Part model, mm, in its own coordinate system. A direction names the side the tool comes from. Coordinates: 2 decimals unless noted, no trailing zeros. Loops run counter-clockwise (first coordinate to the right, second up) from the corner with the lowest first, then second, coordinate; pieces in that order, holes last. Notation, with made-up numbers: (53.5, 42) -> (106.5, 42) arc R4 ccw to (106.5, 46) -> close; hole circle Ø4 at (0, 74.5). An arc over 180 degrees is marked (long way). Use one line per item in the form item = value. Start each with the question number.
(1) Drill centre lines: L1, parallel to Z at x = 0.85, y = 5; L2, parallel to Y at x = 2.6, z = -13 (3 decimals); L3, parallel to Y at x = 0.2, z = -29 (3 decimals). Where is each one in solid material? Low to high. Write a range as [from, to].
(2) Band-saw the part on D-D on y = 43.5. Give the cut face in (x, z) (3 decimals).
(3) Band-saw the part on A-A on z = -14.5. Give the cut face in (x, y) (3 decimals), then the cut area to 3 significant figures.
(4) Band-saw the part on C-C on z = -26. Give the cut face in (x, y) (3 decimals), then the cut area to 3 significant figures.
(5) Pin check, flat tips, straight feed: P1, Ø1, axis at x = 0.5, z = -5, coming from the +Y side; P2, Ø0.9, axis at x = 1, z = -37, coming from the +Y side. Stop position of each tip, or through.
(6) Mould opens along Z. For faces 1 (the flat face through (0, -4, -4)), 2 (the flat face through (2, 12, 0)), 3 (the flat face through (2, -12, -11.5)) say: +Z half, -Z half, draft (parallel to the pull), parting line (faces both ways), or undercut.
(7) 3-axis set-ups, long thin cutter, end or side, ignore diameter. For faces 4 (the flat face through (2, 0, -3)), 5 (the flat face through (2, 10, -37)), 6 (the flat face through (2, 25, -1)), 7 (the flat face through (2, 1, -16.5)): which of +Z, -Z, +X, -X, +Y, -Y reach the whole face in a straight line?
```python
from build123d import *

# Parameters (mm, degrees)
BOSS_EXTRUDE1_DEPTH = 3.175
FILLET1_R           = 1


with BuildPart() as part:
    # Sketch1 → Boss-Extrude1 (new body)
    with BuildSketch(Plane(origin=(0, 0, 0), x_dir=(0, 0, -1), z_dir=(1, 0, 0))):
        with BuildLine():
            Line((6.5, 0), (0, 0))
            Line((0, 0), (0, 25))
            Line((0, 25), (3.5, 25))
            Line((3.5, 25), (0, 35))
            Line((0, 35), (0, 47))
            Line((0, 47), (-8.5, 47))
            Line((-8.5, 47), (-8.5, -25))
            Line((-8.5, -25), (31.5, -25))
            Line((31.5, -25), (31.5, -13.175))
            Line((31.5, -13.175), (11.5, -13.175))
            Line((11.5, -13.175), (11.5, -10))
            Line((11.5, -10), (31.5, -10))
            ThreePointArc((31.5, -10), (37.279601373, -5.967005826), (39.5, 0.721690905))
            Line((39.5, 0.721690905), (39.5, 10))
            Line((39.5, 10), (34.5, 10))
            Line((34.5, 10), (34.5, 0))
            Line((34.5, 0), (16.5, 0))
            Line((16.5, 0), (16.5, 3.5))
            Line((16.5, 3.5), (6.5, 3.5))
            Line((6.5, 3.5), (6.5, 0))
        make_face()
    extrude(amount=BOSS_EXTRUDE1_DEPTH)

    # Fillet1
    fillet1_edges = [part.edges().sort_by_distance(p)[0] for p in [
        (1.5875, -10, -31.5),
        (1.5875, -13.175, -31.5),
        (1.5875, -25, -31.5),
        (1.5875, -25, 8.5),
        (1.5875, 47, 8.5),
        (1.5875, 47, 0),
        (1.5875, 25, -3.5),
        (1.5875, 3.5, -6.5),
        (1.5875, 3.5, -16.5),
        (1.5875, 10, -34.5),
        (1.5875, 10, -39.5),
    ]]
    fillet(fillet1_edges, radius=FILLET1_R)


solid = part.part
```
A:
q1.L1 = [-39.5, -34.5], [0, 8.5]
q1.L2 = [-25, -13.175], [-10, 3.5]
q1.L3 = [-25, -13.175], [-10, 0]
q2.outline = (0, 0) -> (3.175, 0) -> (3.175, 8.5) -> (0, 8.5) -> close
q3.outline = (0, -25) -> (3.175, -25) -> (3.175, -13.175) -> (0, -13.175) -> close; (0, -10) -> (3.175, -10) -> (3.175, 3.5) -> (0, 3.5) -> close
q3.area = 80.4 mm²
q4.outline = (0, -25) -> (3.175, -25) -> (3.175, -13.175) -> (0, -13.175) -> close; (0, -10) -> (3.175, -10) -> (3.175, 0) -> (0, 0) -> close
q4.area = 69.3 mm²
q5.P1 = 0
q5.P2 = 10
q6.face_1 = draft
q6.face_2 = undercut
q6.face_3 = -Z half
q7.face_4 = +X, -X
q7.face_5 = -Z, +X, -X, +Y
q7.face_6 = -Z, +X, -X
q7.face_7 = +X, -X, +Y
